Part model, mm, in its own coordinate system. A direction names the side the tool comes from. Give positions to 0.01 mm unless a question says otherwise; leave off trailing zeros. Loops run counter-clockwise (first coordinate to the right, second up) from the corner with the lowest first, then second, coordinate; pieces in that order, holes last. Notation, with made-up numbers: M 53,-10.5 L 73,-10.5 A15 cw 73,14.5 Z; hole C 0.5,36.25 d10. An arc over 180 degrees is marked long. Answer in a Markdown table with one row per item.
from build123d import *

# Parameters (mm, degrees)
SKETCH1_R                = 200
BOSS_EXTRUDE1_DEPTH      = 15
BOSS_EXTRUDE2_DEPTH      = 200
CUT_EXTRUDE1_DEPTH       = 286.087705803
CUT_EXTRUDE1_DEPTH_BACK  = 286.087705803
SKETCH3_R                = 85
CUT_EXTRUDE2_DEPTH       = 451.079120005
CUT_EXTRUDE2_DEPTH_BACK  = 451.079120005
SKETCH4_R                = 11
CUT_EXTRUDE3_DEPTH       = 451.079120105
CUT_EXTRUDE3_DEPTH_BACK  = 110
CUT_EXTRUDE4_DEPTH       = 110
BOSS_EXTRUDE3_DEPTH      = 200
CUT_EXTRUDE5_DEPTH       = 286.087705815
CUT_EXTRUDE5_DEPTH_BACK  = 286.087705815
SKETCH7_OUTSIDE_W        = 515.59
SKETCH7_OUTSIDE_H        = 515.59
SKETCH7_OUTSIDE_R        = 200
SKETCH9_R                = 4
BOSS_EXTRUDE4_DEPTH      = 220
CUT_EXTRUDE6_DEPTH       = 190
SKETCH11_R               = 3
CUT_EXTRUDE7_DEPTH       = 486.974499745
CUT_EXTRUDE8_DEPTH       = 300.457843596
CUT_EXTRUDE8_DEPTH_BACK  = 300.457843596
SKETCH12_OUTSIDE_W       = 561.36
SKETCH12_OUTSIDE_H       = 521.36
BOSS_EXTRUDE5_DEPTH      = 160
BOSS_EXTRUDE6_DEPTH      = 160
CUT_EXTRUDE9_START       = 15
CUT_EXTRUDE9_DEPTH       = 20
CUT_EXTRUDE10_DEPTH      = 254.564671702
CUT_EXTRUDE10_DEPTH_BACK = 254.564671702
SKETCH17_W               = 10
SKETCH17_H               = 6
CUT_EXTRUDE11_DEPTH      = 221.752620232
CUT_EXTRUDE11_DEPTH_BACK = 221.752620232
SKETCH18_W               = 10
SKETCH18_H               = 6
SKETCH19_R               = 2.75
CUT_EXTRUDE12_DEPTH      = 10
SKETCH20_R               = 2.75
CUT_EXTRUDE13_DEPTH      = 10


# Read off the part's stored shape, not the designer's step: Cut-Extrude9
with BuildPart() as part:
    # Sketch1 → Boss-Extrude1 (new body)
    with BuildSketch(Plane(origin=(0, 0, 0), x_dir=(1, 0, 0), z_dir=(0, 1, 0))):
        with Locations(Location((0, 0, 0), (0, 0, 270))):
            Circle(SKETCH1_R)
    extrude(amount=BOSS_EXTRUDE1_DEPTH)

    # Sketch2 → Boss-Extrude2 (add, symmetric)
    with BuildSketch(Plane.XY):
        Polygon((-25, 50.707142143), (25, 50.707142143), (60, 15), (-60, 15), align=None)
    extrude(amount=BOSS_EXTRUDE2_DEPTH, both=True)

    # Sketch3 → Cut-Extrude1 (cut, two sides: drawn at the far end of the back side and taken through both)
    with BuildSketch(Plane(origin=(0, 15, 0), x_dir=(1, 0, 0), z_dir=(0, 1, 0)).offset(-CUT_EXTRUDE1_DEPTH_BACK)):
        with Locations(Location((0, 0, 0), (0, 0, 270))):
            Circle(SKETCH3_R)
    extrude(amount=CUT_EXTRUDE1_DEPTH + CUT_EXTRUDE1_DEPTH_BACK, mode=Mode.SUBTRACT)

    # Sketch4 → Cut-Extrude2 (cut, two sides: drawn at the far end of the back side and taken through both)
    with BuildSketch(Plane(origin=(0, 0, -200), x_dir=(-1, 0, 0), z_dir=(0, 0, -1)).offset(-CUT_EXTRUDE2_DEPTH_BACK)):
        with Locations((0, 29)):
            Circle(SKETCH4_R)
    extrude(amount=CUT_EXTRUDE2_DEPTH + CUT_EXTRUDE2_DEPTH_BACK, mode=Mode.SUBTRACT)

    # Sketch5 → Cut-Extrude3 (cut, two sides: drawn at the far end of the back side and taken through both)
    with BuildSketch(Plane.XY.offset(200).offset(-CUT_EXTRUDE3_DEPTH_BACK)):
        Polygon((-25, 50.707142143), (25, 50.707142143), (50.198039412, 25), (25, 25), (25, 15), (-25, 15), (-25, 25), (-50.198039412, 25), align=None)
    extrude(amount=CUT_EXTRUDE3_DEPTH + CUT_EXTRUDE3_DEPTH_BACK, mode=Mode.SUBTRACT)

    # Sketch6 → Cut-Extrude4 (cut)
    with BuildSketch(Plane(origin=(0, 0, -200), x_dir=(-1, 0, 0), z_dir=(0, 0, -1))):
        Polygon((-25, 50.707142143), (25, 50.707142143), (50.198039412, 25), (25, 25), (25, 15), (-25, 15), (-25, 25), (-50.198039412, 25), align=None)
    extrude(amount=-CUT_EXTRUDE4_DEPTH, mode=Mode.SUBTRACT)

    # Sketch8 → Boss-Extrude3 (add, symmetric)
    with BuildSketch(Plane(origin=(0, 0, 0), x_dir=(0, 0, -1), z_dir=(1, 0, 0))):
        Polygon((0, 15), (-20, 15), (-10, 35.712315177), (10, 35.712315177), (20, 15), align=None)
    extrude(amount=BOSS_EXTRUDE3_DEPTH, both=True)

    # Sketch7 outside → Cut-Extrude5 (cut, two sides: drawn at the far end of the back side and taken through both)
    with BuildSketch(Plane(origin=(0, 15, 0), x_dir=(1, 0, 0), z_dir=(0, 1, 0)).offset(-CUT_EXTRUDE5_DEPTH_BACK)):
        Rectangle(SKETCH7_OUTSIDE_W, SKETCH7_OUTSIDE_H)
        with Locations(Location((0, 0, 0), (0, 0, 97.180755781))):
            Circle(SKETCH7_OUTSIDE_R, mode=Mode.SUBTRACT)
    extrude(amount=CUT_EXTRUDE5_DEPTH + CUT_EXTRUDE5_DEPTH_BACK, mode=Mode.SUBTRACT)

    # Sketch9 → Boss-Extrude4 (add, symmetric)
    with BuildSketch(Plane(origin=(0, 0, 0), x_dir=(0, 0, -1), z_dir=(1, 0, 0))):
        with Locations(Location((0, 29, 0), (0, 0, 180))):
            Circle(SKETCH9_R)
    extrude(amount=BOSS_EXTRUDE4_DEPTH, both=True)

    # Sketch10 → Cut-Extrude6 (cut, symmetric)
    with BuildSketch(Plane(origin=(0, 0, 0), x_dir=(0, 0, -1), z_dir=(1, 0, 0))):
        Polygon((-20, 15), (20, 15), (10, 35.712315177), (-10, 35.712315177), align=None)
    extrude(amount=CUT_EXTRUDE6_DEPTH, both=True, mode=Mode.SUBTRACT)

    # Sketch11 → Cut-Extrude7 (cut, through all)
    with BuildSketch(Plane.ZY.offset(220)):
        with Locations((0, 29)):
            Circle(SKETCH11_R)
    extrude(amount=-CUT_EXTRUDE7_DEPTH, mode=Mode.SUBTRACT)

    # Sketch12 outside → Cut-Extrude8 (cut, two sides: drawn at the far end of the back side and taken through both)
    with BuildSketch(Plane(origin=(0, 15, 0), x_dir=(1, 0, 0), z_dir=(0, 1, 0)).offset(-CUT_EXTRUDE8_DEPTH_BACK)):
        Rectangle(SKETCH12_OUTSIDE_W, SKETCH12_OUTSIDE_H)
        Polygon((80, 28.722813233), (80, 205.18025718), (287.401401401, 28.722813233), align=None, mode=Mode.SUBTRACT)
    extrude(amount=CUT_EXTRUDE8_DEPTH + CUT_EXTRUDE8_DEPTH_BACK, mode=Mode.SUBTRACT)

    # Sketch13 → Boss-Extrude5 (add)
    with BuildSketch(Plane.XY.offset(-28.722813233)):
        Polygon((80, 15), (80, 35), (90, 35), (90, 25), (99.19, 15), align=None)
    extrude(amount=-BOSS_EXTRUDE5_DEPTH)

    # Sketch15 → Boss-Extrude6 (add)
    with BuildSketch(Plane(origin=(90, 0, 0), x_dir=(0, 0, -1), z_dir=(1, 0, 0))):
        Polygon((28.722813233, 15), (28.722813233, 35), (38.722813233, 35), (38.722813233, 25), (47.915201388, 15), align=None)
    extrude(amount=BOSS_EXTRUDE6_DEPTH)

    # Cut-Extrude9 outline → Cut-Extrude9 (cut)
    with BuildSketch(Plane(origin=(0, 0, 0), x_dir=(1, 0, 0), z_dir=(0, 1, 0)).offset(CUT_EXTRUDE9_START)):
        with BuildLine():
            Line((78, 184.175899359), (80, 183.303027798))
            ThreePointArc((80, 183.303027798), (159.011260133, 121.307127371), (197.926754129, 28.722813233))
            Line((197.926754129, 28.722813233), (250, 28.722813233))
            Line((250, 28.722813233), (250, 188.722813233))
            Line((250, 188.722813233), (78, 188.722813233))
            Line((78, 188.722813233), (78, 184.175899359))
        make_face()
    extrude(amount=CUT_EXTRUDE9_DEPTH, mode=Mode.SUBTRACT)

    # Sketch17 → Cut-Extrude10 (cut, two sides: drawn at the far end of the back side and taken through both)
    with BuildSketch(Plane.XY.offset(-28.722813233).offset(-CUT_EXTRUDE10_DEPTH_BACK)):
        with Locations((85, 7.5)):
            Rectangle(SKETCH17_W, SKETCH17_H)
    extrude(amount=CUT_EXTRUDE10_DEPTH + CUT_EXTRUDE10_DEPTH_BACK, mode=Mode.SUBTRACT)

    # Sketch18 → Cut-Extrude11 (cut, two sides: drawn at the far end of the back side and taken through both)
    with BuildSketch(Plane.ZY.offset(-80).offset(-CUT_EXTRUDE11_DEPTH_BACK)):
        with Locations((-33.722813233, 7.5)):
            Rectangle(SKETCH18_W, SKETCH18_H)
    extrude(amount=CUT_EXTRUDE11_DEPTH + CUT_EXTRUDE11_DEPTH_BACK, mode=Mode.SUBTRACT)

    # Sketch19 → Cut-Extrude12 (cut)
    with BuildSketch(Plane.XY.offset(-28.722813233)):
        with Locations((107.926754129, 30)):
            Circle(SKETCH19_R)
        with Locations((167.926754129, 30)):
            Circle(SKETCH19_R)
        with Locations((137.926754129, 30)):
            Circle(SKETCH19_R)
    extrude(amount=-CUT_EXTRUDE12_DEPTH, mode=Mode.SUBTRACT)

    # Sketch20 → Cut-Extrude13 (cut)
    with BuildSketch(Plane.ZY.offset(-80)):
        with Locations((-163.303027798, 30)):
            Circle(SKETCH20_R)
        with Locations((-133.303027798, 30)):
            Circle(SKETCH20_R)
        with Locations((-103.303027798, 30)):
            Circle(SKETCH20_R)
    extrude(amount=-CUT_EXTRUDE13_DEPTH, mode=Mode.SUBTRACT)


solid = part.part
(1) Pull direction X, two halves, no side cores. Call faces 1 (the face through (139.405, 32.319, -33.653)), 2 (the face through (94.53, 20.07, -107.69)), 3 (the face through (140, 2, -28.723)), 4 (the face through (80, 23, -105)): +X half, -X half, draft (parallel to the pull), parting line (faces both ways), or undercut.
Recorded:
| item | result |
|---|---|
| face 1 | undercut |
| face 2 | +X half |
| face 3 | draft |
| face 4 | -X half |
(2) Saw through at A-A (y = 30). Give the number of separate pieces and of enclosed holes in the cut face, plus the area to 3 significant figures.
Recorded:
| item | result |
|---|---|
| separate pieces | 7 |
| enclosed holes | 0 |
| area | 2,260 mm^2 |
(3) Saw through at B-B (z = -164). Write the cut outline in (x, y), plus the area to 3 significant figures.
Recorded:
| item | result |
|---|---|
| outline | M 80,0 L 114.47,0 L 114.47,15 L 99.19,15 L 90,25 L 90,27.34 L 80,27.34 L 80,10.5 L 90,10.5 L 90,4.5 L 80,4.5 Z; M 80,32.66 L 90,32.66 L 90,35 L 80,35 Z |
| area | 650 mm^2 |
(4) Saw through at D-D (x = 176). Write the cut outline in (y, z), plus the area to 3 significant figures.
Recorded:
| item | result |
|---|---|
| outline | M 0,-94.99 L 15,-94.99 L 15,-47.92 L 25,-38.72 L 35,-38.72 L 35,-28.72 L 10.5,-28.72 L 10.5,-38.72 L 4.5,-38.72 L 4.5,-28.72 L 0,-28.72 Z |
| area | 1,180 mm^2 |
(5) Pin check, flat tips, straight feed: pin 1 Ø6.5 at (x, y) = (139, 8.5) entering from +Z; pin 2 Ø5 at (x, y) = (107.93, 30) entering from +Z; pin 3 Ø3 at (x, y) = (131, 31) entering from -Z; pin 4 Ø5 at (y, z) = (8, -110.5) entering from +X. Stop position of each tip, or through.
Recorded:
| item | result |
|---|---|
| pin 1 | stops at z = -28.72 |
| pin 2 | passes through |
| pin 3 | stops at z = -38.72 |
| pin 4 | stops at x = 168.33 |
(6) Which spindle directions (+Z, -Z, +X, -X, +Y, -Y) get a long thin tool onto all of the face, cutting with end or side? Do faces 5 (the face through (86, 10.5, -72)), 6 (the face through (144, 7, -38.723)), 7 (the face through (142, 30, -38.723)). Say none if no direction does.
Recorded:
| item | result |
|---|---|
| face 5 | +Z, -X |
| face 6 | +Z, +X, -X |
| face 7 | -Z, +X, +Y |
(7) Saw through at C-C (z = -121.5). Write the cut outline in (x, y).
Recorded:
| item | result |
|---|---|
| outline | M 80,0 L 158.86,0 L 158.86,15 L 99.19,15 L 90,25 L 90,35 L 80,35 L 80,10.5 L 90,10.5 L 90,4.5 L 80,4.5 Z |
(8) Drill centre lines: line 1 along Z through (x, y) = (152.5, 30); line 2 along Y through (x, z) = (101.5, -106); line 3 along Z through (x, y) = (90, 21). Where is each one in solid material? Low to high.
Recorded:
| item | result |
|---|---|
| line 1 | z = -38.72 to -28.72 |
| line 2 | y = 0 to 15 |
| line 3 | z = -178.61 to -28.72 |
